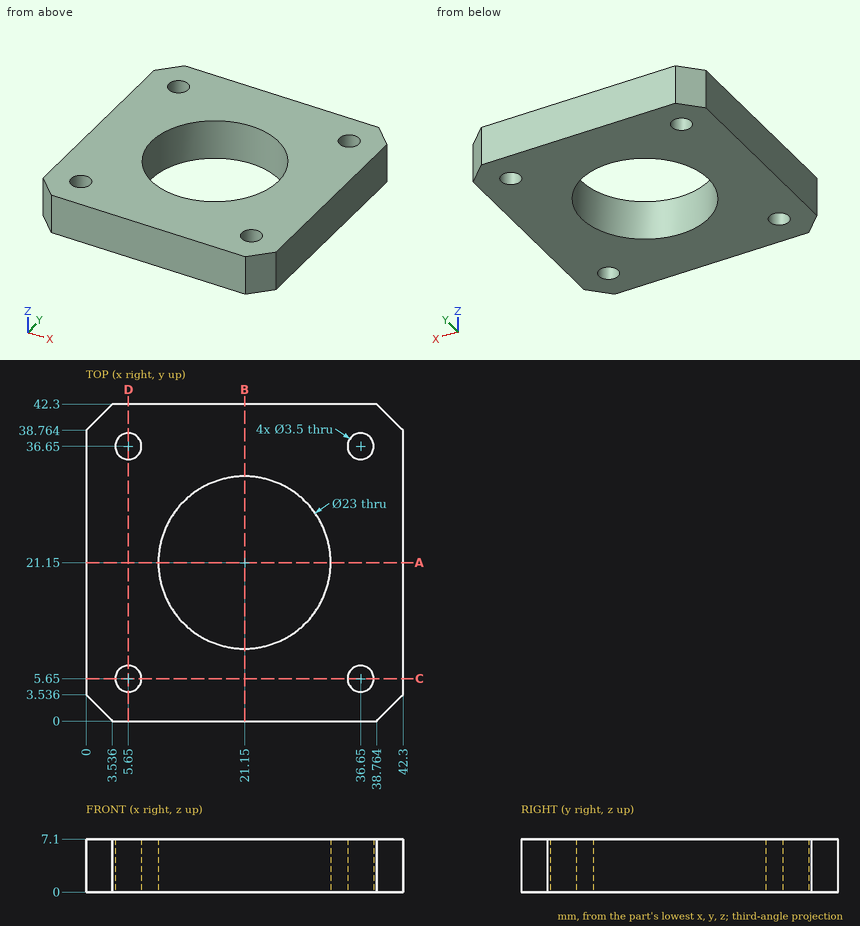
The drawing under review shows one solid part. Ordinate dimensions are in mm from its lowest x, y, z. Coordinates: 2 decimals unless noted, no trailing zeros. Write each loop counter-clockwise with the first axis right and the second up, starting at its lowest first coordinate (ties: lowest second). Pieces come first, ordered by that corner, then holes. Notation, with made-up numbers: (-28, -27.5) -> (21, -27.5) arc R16 cw to (21, -15.5) -> close; hole circle Ø2 at (18.25, 18). An arc over 180 degrees is marked (long way). Write each question's results on one line, items separated by ' | '. Start each with the question number.
1) Consider section C-C (y = 5.65). Write out the cut boundary in (x, z).
2) Insertion check: pin 1 (4.5 mm diameter, centred on x = 5.65, y = 5.65, fed in from -Z). The pin has a flat end and moves straight along its axis. Give the tip position at first contact, or say it passes through.
3) Consider section A-A (y = 21.15). Write out the cut boundary in (x, z).
4) Wall thickness on L1, parallel to Y at x = 5.65, z = 5.25; L2, parallel to Y at x = 21.15, z = 2.25; L3, parallel to Y at x = 14, z = 3.5 (1 decimal): over which ranges is each line inside the solid? List them lowest first. Write a range as [from, to].
Geometry says:
1) outline: (0, 0) -> (3.9, 0) -> (3.9, 7.1) -> (0, 7.1) -> close; (7.4, 0) -> (34.9, 0) -> (34.9, 7.1) -> (7.4, 7.1) -> close; (38.4, 0) -> (42.3, 0) -> (42.3, 7.1) -> (38.4, 7.1) -> close
2) pin 1: z = 0
3) outline: (0, 0) -> (9.65, 0) -> (9.65, 7.1) -> (0, 7.1) -> close; (32.65, 0) -> (42.3, 0) -> (42.3, 7.1) -> (32.65, 7.1) -> close
4) L1: [0, 3.9], [7.4, 34.9], [38.4, 42.3] | L2: [0, 9.65], [32.65, 42.3] | L3: [0, 12.1], [30.2, 42.3]
